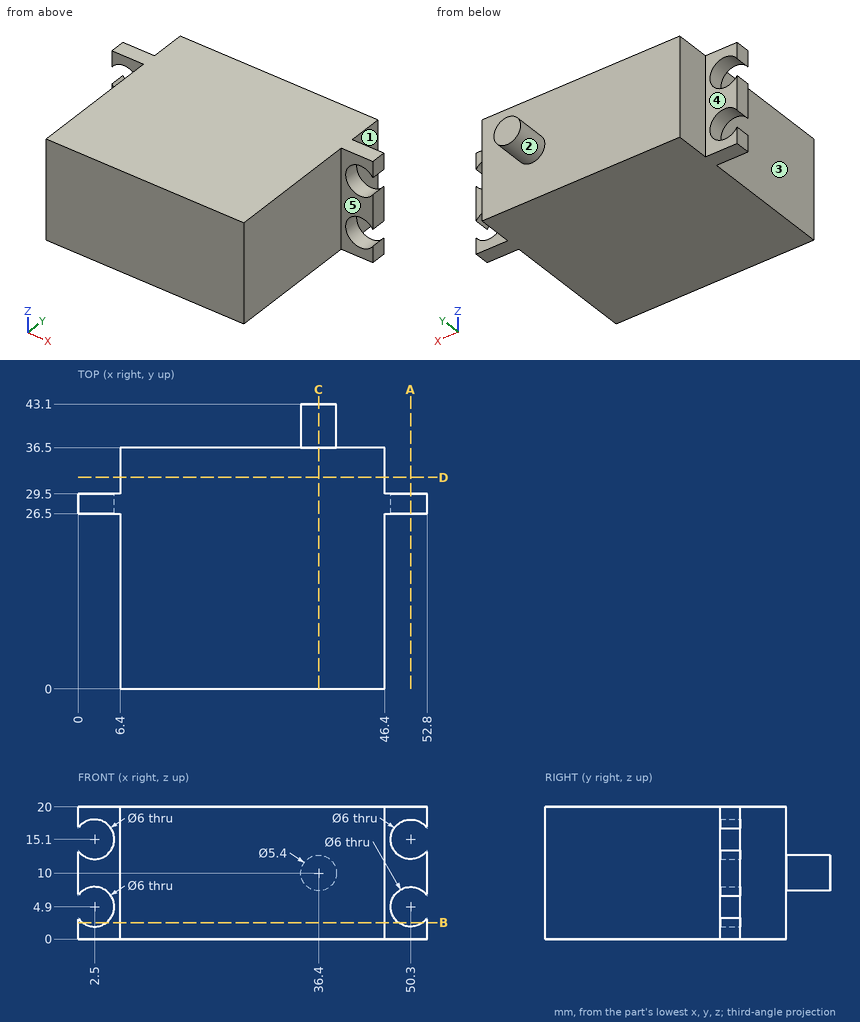
Job drawing, mm, ordinate dimensions from the low corner. One solid piece. A direction names the side the tool comes from. Give positions to 0.01 mm unless a question says otherwise; leave off trailing zeros. Write each loop counter-clockwise with the first axis right and the second up, starting at its lowest first coordinate (ties: lowest second). Pieces come first, ordered by that corner, then holes. Notation, with made-up numbers: (78, 33) - (119, 33) arc R15 ccw to (119, 41) - close; hole circle Ø1 at (-27, 17.5). An arc over 180 degrees is marked (long way). Use one line per item in the form item = value. Start each with the question number.
1. Band-saw the part on D-D on y = 32. Write the cut outline in (x, z).
2. 3-axis set-ups, long thin cutter, end or side, ignore diameter. For the marked faces 1, 2, 3, 4 and 5: which of +Z, -Z, +X, -X, +Y, -Y reach the whole face in a straight line?
3. Band-saw the part on C-C on x = 36.4. Write the cut outline in (y, z), plus the area to 3 significant figures.
4. Probe line 1 (Z direction, x = 2.5, y = 27.85); line 2 (X direction, y = 28.75, z = 4.9); line 3 (Y direction, x = 31, z = 3). List the from-to ranges inside material, lowest first. Write a range as [from, to].
5. Drop flat-ended pins along their axis: pin 1 Ø1.9 at (x, z) = (48.5, 12) entering from -Y; pin 2 Ø2 at (y, z) = (35, 5.5) entering from +X; pin 3 Ø1.5 at (y, z) = (13.5, 17) entering from -X. Give the stop position or say it passes through.
6. Band-saw the part on A-A on x = 50.3. Write the cut outline in (y, z), plus the area to 3 significant figures.
7. Band-saw the part on B-B on z = 2.5. Write the cut outline in (x, y), plus the area to 3 significant figures.
Conclusion:
q1.outline = (6.4, 0) - (46.4, 0) - (46.4, 20) - (6.4, 20) - close
q2.face_1 = +Z, -Z, +X, +Y
q2.face_2 = +Y
q2.face_3 = +Z, -Z, -X, -Y
q2.face_4 = +Z, -Z, -X, +Y
q2.face_5 = +Z, -Z, +X, -Y
q3.outline = (0, 0) - (36.5, 0) - (36.5, 7.3) - (43.1, 7.3) - (43.1, 12.7) - (36.5, 12.7) - (36.5, 20) - (0, 20) - close
q3.area = 766 mm²
q4.line_1 = [0, 1.9], [7.9, 12.1], [18.1, 20]
q4.line_2 = [5.5, 47.3]
q4.line_3 = [0, 36.5]
q5.pin_1 = 26.5
q5.pin_2 = 46.4
q5.pin_3 = 6.4
q6.outline = (26.5, 0) - (29.5, 0) - (29.5, 1.9) - (26.5, 1.9) - close; (26.5, 7.9) - (29.5, 7.9) - (29.5, 12.1) - (26.5, 12.1) - close; (26.5, 18.1) - (29.5, 18.1) - (29.5, 20) - (26.5, 20) - close
q6.area = 24.0 mm²
q7.outline = (0, 26.5) - (0.7, 26.5) - (0.7, 29.5) - (0, 29.5) - close; (4.3, 26.5) - (6.4, 26.5) - (6.4, 0) - (46.4, 0) - (46.4, 26.5) - (48.5, 26.5) - (48.5, 29.5) - (46.4, 29.5) - (46.4, 36.5) - (6.4, 36.5) - (6.4, 29.5) - (4.3, 29.5) - close; (52.1, 26.5) - (52.8, 26.5) - (52.8, 29.5) - (52.1, 29.5) - close
q7.area = 1,480 mm²
